Could you check a few things on this model? Use its own coordinates, in mm. A direction names the side the tool comes from. Coordinates: 2 decimals unless noted, no trailing zeros. Write each loop counter-clockwise with the first axis right and the second up, starting at its lowest first coordinate (ties: lowest second). Pieces come first, ordered by that corner, then holes. Notation, with made-up numbers: M 9.25,-2 L 30.25,-2 A8 ccw 30.25,12 Z; hole C 37,29 d5. An arc over 180 degrees is marked long. Write item = value, one per line.
```python
from build123d import *

# Parameters (mm, degrees)
BOSS_EXTRUDE1_DEPTH = 6.35
SKETCH2_W           = 6.35
SKETCH2_H           = 15.306086647
CUT_EXTRUDE1_DEPTH  = 281.120661501


with BuildPart() as part:
    # Sketch1 → Boss-Extrude1 (new body)
    with BuildSketch(Plane.XY):
        with BuildLine():
            Line((0, 0), (19.05, 0))
            Line((19.05, 0), (19.05, 12.7))
            Line((19.05, 12.7), (0, 12.7))
            Line((0, 12.7), (0, 19.05))
            Line((0, 19.05), (19.05, 19.05))
            ThreePointArc((19.05, 19.05), (22.75701822, 18.530813768), (26.178773585, 17.013207547))
            ThreePointArc((26.178773585, 17.013207547), (27.935718963, 15.16706609), (28.575, 12.7))
            Line((28.575, 12.7), (28.575, 0))
            Line((28.575, 0), (28.575, -3.175))
            Line((28.575, -3.175), (34.925, -3.175))
            Line((34.925, -3.175), (34.925, 12.131086647))
            Line((34.925, 12.131086647), (139.7, 12.131086647))
            Line((139.7, 12.131086647), (139.7, -13.843))
            Line((139.7, -13.843), (0, -13.843))
            Line((0, -13.843), (0, 0))
        make_face()
    boss_extrude1 = extrude(amount=BOSS_EXTRUDE1_DEPTH)

    # Mirror1: Boss-Extrude1 across plane
    add(boss_extrude1.mirror(Plane(origin=(139.7, 12.131086647, 6.35), x_dir=(0, 0, 1), z_dir=(-1, 0, 0))))

    # Sketch2 → Cut-Extrude1 (cut, through all)
    with BuildSketch(Plane.XY.offset(6.35)):
        with Locations((103.716666667, 4.478043323)):
            Rectangle(SKETCH2_W, SKETCH2_H)
        with Locations((175.683333333, 4.478043323)):
            Rectangle(SKETCH2_W, SKETCH2_H)
    extrude(amount=-CUT_EXTRUDE1_DEPTH, mode=Mode.SUBTRACT)


solid = part.part
```
Item 1: If we mould it in two halves opening along Y, with no side actions, what happens to faces 1 (the face through (0, 16, 3)), 2 (the face through (138, -13.843, 3)), 3 (the face through (19.05, 6, 3))? For each: pulls with the +Y half, pulls with the -Y half, needs draft (parallel to the pull), parting line crosses it, or undercut.
Numbers:
face_1 = needs draft
face_2 = pulls with the -Y half
face_3 = undercut
Item 2: Imagine slicing it at C-C (x = 213.5). Write out the boundary of the cut face in (y, z).
Numbers:
outline = M -13.84,0 L 12.13,0 L 12.13,6.35 L -13.84,6.35 Z
Item 3: For faces 4 (the face through (140, 12.131, 3)), 5 (the face through (260.35, 6, 3)), 6 (the face through (138, -1, 0)), which set-ups out of +Z, -Z, +X, -X, +Y, -Y let a thin tool reach every point of the face, with its end or its side?
Numbers:
face_4 = +Z, -Z, +Y
face_5 = +Z, -Z, +X
face_6 = -Z, +X, -X, +Y, -Y
Item 4: Imagine slicing it at A-A (y = 8.5). Write out the boundary of the cut face in (x, z) (3 decimals), and give its area (3 significant figures).
Numbers:
outline = M 19.05,0 L 28.575,0 L 28.575,6.35 L 19.05,6.35 Z; M 34.925,0 L 100.542,0 L 100.542,6.35 L 34.925,6.35 Z; M 106.892,0 L 172.508,0 L 172.508,6.35 L 106.892,6.35 Z; M 178.858,0 L 244.475,0 L 244.475,6.35 L 178.858,6.35 Z; M 250.825,0 L 260.35,0 L 260.35,6.35 L 250.825,6.35 Z
area = 1,370 mm²
Item 5: I'm going to push flat-ended pins straight in: P1, Ø3, axis at x = 77.5, z = 1, coming from the +Y side; P2, Ø3, axis at x = 175, z = 4.5, coming from the +Y side (3 decimals); P3, Ø3, axis at y = 4.5, z = 4, coming from the +X side. Where does each tip first touch, or does it pass through?
Numbers:
P1 = 12.13
P2 = -3.175
P3 = 260.35
Item 6: If I drill on line 1 along X through (y, z) = (-0.5, 4.5) (3 decimals); line 2 along X through (y, z) = (10, 6) (3 decimals); line 3 along Y through (x, z) = (262.5, 3.5), over which ranges is the centre line in solid material (lowest first)?
Numbers:
line_1 = 0 to 28.575, 34.925 to 100.542, 106.892 to 172.508, 178.858 to 244.475, 250.825 to 279.4
line_2 = 19.05 to 28.575, 34.925 to 100.542, 106.892 to 172.508, 178.858 to 244.475, 250.825 to 260.35
line_3 = -13.84 to 0, 12.7 to 19.05
Item 7: Imagine slicing it at D-D (x = 32). Write out the boundary of the cut face in (y, z) (3 decimals), and give its area (3 significant figures).
Numbers:
outline = M -13.843,0 L -3.175,0 L -3.175,6.35 L -13.843,6.35 Z
area = 67.7 mm²
